from build123d import *

# Parameters (mm, degrees)
F1_DEPTH = 8
F2_T     = -2
F3_R     = 2
F4_R     = 2


with BuildPart() as f1:
    # F0 (on Top) → F1 (new body)
    with BuildSketch(Plane.XY):
        with BuildLine():
            ThreePointArc((-85, -31), (-82.3639610307, -37.3639610307), (-76, -40))
            Line((-76, -40), (76, -40))
            ThreePointArc((76, -40), (82.3639610307, -37.3639610307), (85, -31))
            Line((85, -31), (85, 31))
            ThreePointArc((85, 31), (82.3639610307, 37.3639610307), (76, 40))
            Line((76, 40), (-76, 40))
            ThreePointArc((-76, 40), (-82.3639610307, 37.3639610307), (-85, 31))
            Line((-85, 31), (-85, -31))
        make_face()
    extrude(amount=F1_DEPTH)

    # F2
    f2_openings = [f1.faces().sort_by_distance(p)[0] for p in [
        (0, 0, 8),
    ]]
    offset(amount=F2_T, openings=f2_openings)

    # F3
    f3_edges = [f1.edges().sort_by_distance(p)[0] for p in [
        (0, 38, 2),
    ]]
    fillet(f3_edges, radius=F3_R)

    # F4
    f4_edges = [f1.edges().sort_by_distance(p)[0] for p in [
        (0, -40, 0),
    ]]
    fillet(f4_edges, radius=F4_R)


solid = f1.part
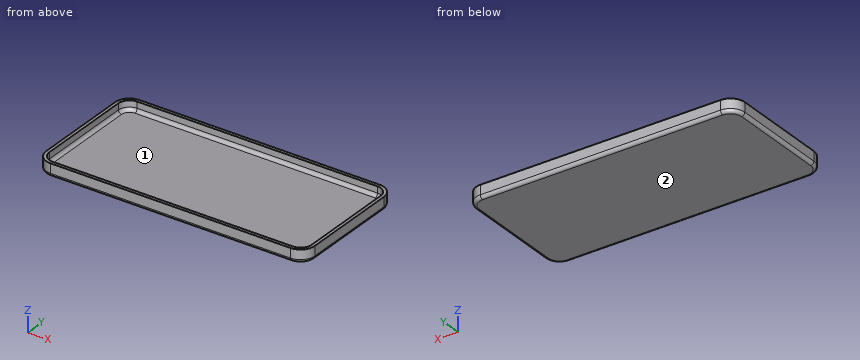
For this review, take the finished solid that the model builds, in its own axes (mm). Face numbers are marked on the shaded views. Give positions to 0.01 mm unless a question says otherwise; leave off trailing zeros. Loops run counter-clockwise (first coordinate to the right, second up) from the corner with the lowest first, then second, coordinate; pieces in that order, holes last. Notation, with made-up numbers: M 33.25,-29.5 L 86.25,-29.5 A24 ccw 86.25,0.5 Z; hole C 39,73 d2. An arc over 180 degrees is marked long. Put each result on its own line as item: value. Start each with the question number.
(1) Add section C-C, the plane x = -5. Write out the cut boundary in (y, z), then the cut area to 3 significant figures.
(2) For pin 1 (3 mm diameter, centred on x = 67.5, y = -5, fed in from +Z), flat-tipped, find the tip position at first contact; note if it passes through.
(3) Add section A-A, the plane z = 6.25. Write out the cut boundary in (x, y), then the cut area to 3 significant figures.
(4) The part is to be moulded in two halves that separate along X. For the marked faces 1 and 2, say which applies: +X half, -X half, draft (parallel to the pull), parting line (faces both ways), or undercut.
(5) Wall thickness on L1, parallel to Y at x = -75, z = 4.5; L2, parallel to X at y = 18, z = 7.25; L3, parallel to Z at x = -40, y = 3: over which ranges is each line inside the solid? List them lowest first.
(6) Add section B-B, the plane y = -3.5. Write out the cut boundary in (x, z), then the cut area to 3 significant figures.
Result:
1. outline: M -40,2 A2 ccw -38,0 L 38,0 A2 ccw 40,2 L 40,8 L 38,8 L 38,4 A2 cw 36,2 L -36,2 A2 cw -38,4 L -38,8 L -40,8 Z
1. area: 184 mm^2
2. pin 1: stops at z = 2
3. outline: M -85,-31 A9 ccw -76,-40 L 76,-40 A9 ccw 85,-31 L 85,31 A9 ccw 76,40 L -76,40 A9 ccw -85,31 Z; hole M -83,-31 A7 ccw -76,-38 L 76,-38 A7 ccw 83,-31 L 83,31 A7 ccw 76,38 L -76,38 A7 ccw -83,31 Z
3. area: 957 mm^2
4. face 1: undercut
4. face 2: draft
5. L1: y = -40 to -38, 38 to 40
5. L2: x = -85 to -83, 83 to 85
5. L3: z = 0 to 2
6. outline: M -85,2 A2 ccw -83,0 L 83,0 A2 ccw 85,2 L 85,8 L 83,8 L 83,4 A2 cw 81,2 L -81,2 A2 cw -83,4 L -83,8 L -85,8 Z
6. area: 364 mm^2
